```python
from build123d import *

# Parameters (mm, degrees)
F0_W     = 50.8
F0_H     = 50.8
F1_DEPTH = 50.8
F2_SIZE  = 3.175
F3_W     = 19.05
F3_H     = 17.018
F5_W     = 2.1082
F5_H     = 2.1082
F6_DEPTH = 1.0541


with BuildPart() as f1:
    # F0 (on Top) → F1 (new body)
    with BuildSketch(Plane.XY):
        Rectangle(F0_W, F0_H)
    extrude(amount=F1_DEPTH)

    # F2
    f2_edges = [f1.edges().sort_by_distance(p)[0] for p in [
        (25.4, -25.4, 25.4),
        (25.4, 25.4, 25.4),
        (-25.4, 25.4, 25.4),
        (-25.4, -25.4, 25.4),
    ]]
    chamfer(f2_edges, length=F2_SIZE)

    # F3 (on Front) → F4 (revolve)
    with BuildSketch(Plane.XZ):
        with Locations((-9.525, 59.309)):
            Rectangle(F3_W, F3_H)
        with BuildLine():
            Line((-19.05, 67.818), (0, 67.818))
            Line((0, 67.818), (0, 86.4012725589))
            Line((0, 86.4012725589), (-4.191, 86.4012725589))
            ThreePointArc((-4.191, 86.4012725589), (-14.8785256326, 79.7147211869), (-19.05, 67.818))
        make_face()
        Polygon((-4.191, 86.4012725589), (0, 86.4012725589), (0, 86.868), (0, 98.425), (-4.191, 98.425), align=None)
    revolve(axis=Axis((0, 0, 59.309), (0, 0, 1)))

    # F5 (on Front) → F6 (join, symmetric)
    with BuildSketch(Plane.XZ):
        with Locations((-2.1082, 107.9627)):
            Rectangle(F5_W, F5_H)
        Polygon((-1.0541, 98.425), (0, 98.425), (0, 111.125), (-1.0541, 111.125), (-1.0541, 109.0168), (-1.0541, 106.9086), align=None)
    extrude(amount=F6_DEPTH, both=True)

    # F7: F1 across face


with BuildPart() as f1_1:
    add(f1.part)
    add(f1.part.mirror(Plane(origin=(0, 0, 104.775), x_dir=(0, 1, 0), z_dir=(1, 0, 0))))


solid = f1_1.part
```
Geometry check sheet. Reference: the model listing, model coordinates, mm. A direction names the side the tool comes from. Coordinates: 2 decimals unless noted, no trailing zeros. Order: outer loops, then holes, each group sorted by start corner. A loop starts at its lowest first (then second) coordinate and runs counter-clockwise, first axis right, second up. Notation, with made-up numbers: (50.5, 59) - (66.5, 59) arc R20 cw to (66.5, 98) - close; hole circle Ø7 at (29, 72). An arc over 180 degrees is marked (long way). Answer as a JSON object with one key per item and string values. Group by question number.
Item 1: Tool access check on faces 4 (the face through (0, 1.054, 105)), 5 (the face through (1.054, 0, 110)), 6 (the face through (-1.054, 0, 103)), 7 (the face through (-3.997, -1.259, 92.329)), 8 (the face through (-1.054, 0, 110)). Record the directions out of +Z, -Z, +X, -X, +Y, -Y that give a thin tool (end or side, any length) a straight path to the whole face; none if there is none.
Item 2: Sectioned sample at D-D, the plane z = 94. Record the cut outline in (x, y).
Item 3: Scan lines: probe 1 along Z at (x, y) = (14, 23.5); probe 2 along X at (y, z) = (0.5, 55); probe 3 along Z at (x, y) = (2.5, -2) (3 decimals). Record each from-to range of solid material in increasing order.
Item 4: Depth check by flat-ended pin: pin 1 Ø1.9 at (x, z) = (0, 107) entering from -Y; pin 2 Ø2 at (x, y) = (-20, -5) entering from +Z; pin 3 Ø8 at (x, y) = (-10.5, 18.5) entering from +Z; pin 4 Ø1.5 at (x, y) = (9.5, 9.5) entering from -Z. Enter the tip coordinate at first touch or a pass-through.
Item 5: Sectioned sample at C-C, the plane y = -17. Record the cut outline in (x, z).
Item 6: Draft check along Z on faces 1 (the face through (-2, 0, 109.017)), 2 (the face through (2, 0, 98.425)), 3 (the face through (0, -1.054, 105)). Enter one of: +Z half, -Z half, draft (parallel to the pull), parting line (faces both ways), or undercut.
Item 7: Sectioned sample at A-A, the plane z = 52.5. Record the cut outline in (x, y).
Item 8: Sectioned sample at B-B, the plane x = -12. Record the cut outline in (y, z), and give its area (3 significant figures).
Resolved:
{
 "1": {"face 4": "+Z, +X, -X, +Y", "face 5": "+Z, +X, +Y, -Y", "face 6": "-X, +Y, -Y", "face 7": "+Z", "face 8": "+Z, -X, +Y, -Y"},
 "2": {"outline": "circle Ø8.38 at (0, 0)"},
 "3": {"probe 1": "0 to 50.8", "probe 2": "-19.04 to 19.04", "probe 3": "0 to 98.425"},
 "4": {"pin 1": "y = -1.05", "pin 2": "z = 50.8", "pin 3": "z = 75.85", "pin 4": "z = 0"},
 "5": {"outline": "(-25.4, 0) - (25.4, 0) - (25.4, 50.8) - (8.6, 50.8) - (8.6, 67.82) arc R8.6 ccw to (-8.6, 67.82) - (-8.6, 50.8) - (-25.4, 50.8) - close"},
 "6": {"face 1": "+Z half", "face 2": "undercut", "face 3": "draft"},
 "7": {"outline": "circle Ø38.1 at (0, 0)"},
 "8": {"outline": "(-25.4, 0) - (25.4, 0) - (25.4, 50.8) - (14.8, 50.8) - (14.8, 67.82) arc R14.8 ccw to (-14.8, 67.82) - (-14.8, 50.8) - (-25.4, 50.8) - close", "area": "3,430 mm^2"}
}
